Verification items for the finished model (mm, model axes). A direction names the side the tool comes from. Coordinates: 2 decimals unless noted, no trailing zeros. Loops run counter-clockwise (first coordinate to the right, second up) from the corner with the lowest first, then second, coordinate; pieces in that order, holes last. Notation, with made-up numbers: (31.5, 79.5) -> (83.5, 79.5) arc R17 cw to (83.5, 99.5) -> close; hole circle Ø4 at (-18, 59.25). An arc over 180 degrees is marked (long way). Write item = value, one per line.
```python
from build123d import *

# Parameters (mm, degrees)
BOSS_EXTRUDE1_DEPTH        = 10
CUT_EXTRUDE1_DEPTH         = 5
F_3_1_3_1_DIAMETER_HOLE2_D = 3.1
BOSS_EXTRUDE2_DEPTH        = 10
FILLET1_R                  = 3
FILLET2_R                  = 2
CUT_EXTRUDE6_DEPTH         = 2.5
SKETCH28_R                 = 3.5000000000000004
CUT_EXTRUDE7_DEPTH         = 2.5
SKETCH29_W                 = 2.5
SKETCH29_H                 = 3.5000000000000004
SKETCH30_R                 = 2.5000000000000004
CUT_EXTRUDE8_DEPTH         = 7.029807515


with BuildPart() as part:
    # Sketch1 → Boss-Extrude1 (new body)
    with BuildSketch(Plane(origin=(0, 0, 0), x_dir=(1, 0, 0), z_dir=(0, 1, 0))):
        with BuildLine():
            ThreePointArc((-207.41455152497886, 32.851237658448525), (-209.99999999999994, 2.572e-14), (-207.41455152497886, -32.85123765844857))
            Line((-207.41455152497886, -32.85123765844857), (-217.29143493093028, -34.41558230885091))
            ThreePointArc((-217.29143493093028, -34.41558230885091), (-220, 2.694e-14), (-217.29143493093028, 34.415582308850865))
            Line((-217.29143493093028, 34.415582308850865), (-207.41455152497886, 32.851237658448525))
        make_face()
        with BuildLine():
            ThreePointArc((-217.2914349309303, -34.415582308850915), (-219.99999999999997, -1.421e-14), (-217.2914349309303, 34.415582308850865))
            Line((-217.29143493093028, 34.41558230885082), (-219.26681161212053, 34.72845123893128))
            ThreePointArc((-219.26681161212053, 34.72845123893128), (-221.99999999999997, -2.665e-14), (-219.26681161212053, -34.72845123893134))
            Line((-219.26681161212053, -34.728451238931335), (-217.29143493093028, -34.41558230885088))
        make_face()
        with BuildLine():
            Line((-205.4391748437886, 32.538368728368056), (-207.41455152497886, 32.85123765844851))
            ThreePointArc((-207.41455152497886, 32.851237658448525), (-209.99999999999994, -2.132e-14), (-207.41455152497886, -32.85123765844859))
            Line((-207.41455152497886, -32.85123765844857), (-205.4391748437886, -32.53836872836811))
            ThreePointArc((-205.43917484378863, -32.53836872836813), (-207.99999999999997, -2.842e-14), (-205.43917484378863, 32.538368728368056))
        make_face()
    extrude(amount=BOSS_EXTRUDE1_DEPTH)

    # Sketch15 → Cut-Extrude1 (cut)
    with BuildSketch(Plane(origin=(0, 10, 0), x_dir=(1, 0, 0), z_dir=(0, 1, 0))):
        with BuildLine():
            Line((-219.7726097583591, 9.999999999999972), (-209.76176963403066, 9.999999999999972))
            ThreePointArc((-209.76176963403046, 9.999999999995824), (-208.90085088283388, 21.457737542154447), (-207.41455152497886, 32.851237658448504))
            Line((-207.41455152497886, 32.851237658448504), (-217.29143493093028, 34.41558230885091))
            ThreePointArc((-217.2914349309303, 34.41558230885091), (-218.8727368927212, 22.242415450882426), (-219.7726097583591, 10.000000000000421))
        make_face()
        with BuildLine():
            ThreePointArc((-207.4145515249789, -32.85123765844855), (-208.90085088283385, -21.457737542154504), (-209.76176963403046, -9.999999999995891))
            Line((-209.76176963403066, -10.000000000000028), (-219.77260975835907, -10.00000000000003))
            ThreePointArc((-219.7726097583591, -10.000000000000506), (-218.8727368927212, -22.242415450882447), (-217.2914349309303, -34.41558230885088))
            Line((-217.29143493093028, -34.41558230885086), (-207.41455152497886, -32.85123765844855))
        make_face()
    extrude(amount=-CUT_EXTRUDE1_DEPTH, mode=Mode.SUBTRACT)

    # Ø3.1 (3.1) Diameter Hole2 (through all)
    with Locations(Plane(origin=(0, 0, 0), x_dir=(-1, 0, 0), z_dir=(0, -1, 0))):
        with Locations((213.160645195, -28.063131327), (214.18186009, -18.738484691), (214.18186009, 18.738484691), (213.160645195, 28.063131327)):
            Hole(F_3_1_3_1_DIAMETER_HOLE2_D / 2)

    # Sketch19 → Boss-Extrude2 (add)
    with BuildSketch(Plane(origin=(0, 0, 0), x_dir=(1, 0, 0), z_dir=(0, 1, 0))):
        with BuildLine():
            Line((-205.06000872553298, -13.44034305679455), (-207.55465603362947, -13.603850879869908))
            ThreePointArc((-207.55465603362947, -13.603850879869908), (-207.99999999999994, 2.547e-14), (-207.55465603362947, 13.603850879869857))
            Line((-207.55465603362947, 13.603850879869857), (-205.06000872553298, 13.440343056794502))
            ThreePointArc((-205.06000872553298, 13.440343056794502), (-205.49999999999997, 2.517e-14), (-205.06000872553298, -13.44034305679455))
        make_face()
    extrude(amount=BOSS_EXTRUDE2_DEPTH)

    # Fillet1
    # the kernel refuses this fillet: 3 mm, written as the material it adds along each edge
    with BuildSketch(Plane(origin=(-207.5546560336295, 0, -13.60385087986986), x_dir=(0.07259195171826252, 0, -0.9973617240228008), z_dir=(0, 1, 0))) as fillet1_piece_1:
        with BuildLine():
            CenterArc((2.97605695844059, -2.9999221104362666), FILLET1_R, 89.58712595875737, 80.81905726138756)
            Line((0.01801487263020066, -2.4999350920302814), (-0.04114596908600657, -2.489935351662162))
            ThreePointArc((-0.04114596908600657, -2.489935351662162), (-0.05099100589383556, -1.2503999029582549), (-0.05999844220872477, -0.00043235694312724))
            Line((-0.05999844220872477, -0.00043235694312724), (-0.00043235694311419, 0.05999844220871681))
            ThreePointArc((-0.00043235694311419, 0.05999844220871681), (1.4988374027981592, 0.06540034308590705), (2.998107162539448, 0.05999844220873665))
            Line((2.998107162539448, 0.05999844220873665), (2.9976748055963345, 1e-17))
        make_face()
    extrude(amount=10)
    with BuildSketch(Plane(origin=(-207.5546560336295, 0, 13.60385087986991), x_dir=(0.07259195171826295, 0, 0.9973617240228008), z_dir=(0, 1, 0))) as fillet1_piece_2:
        with BuildLine():
            CenterArc((2.9760569584405734, 2.9999221104362666), FILLET1_R, 189.5938167798556, 80.819057261387)
            Line((0.01801487263018374, 2.4999350920302543), (-0.04114596908602352, 2.4899353516621354))
            ThreePointArc((-0.04114596908602352, 2.4899353516621354), (-0.05099100589383325, 1.2503999029582546), (-0.05999844220872477, 0.00043235694312726))
            Line((-0.05999844220872477, 0.00043235694312726), (-0.00043235694311422, -0.05999844220871681))
            ThreePointArc((-0.00043235694311422, -0.05999844220871681), (1.498837402798161, -0.06540034308590782), (2.9981071625394304, -0.05999844220873665))
            Line((2.9981071625394304, -0.05999844220873665), (2.9976748055963167, 0))
        make_face()
    extrude(amount=10)

    # Fillet2
    fillet2_edges = [part.edges().sort_by_distance(p)[0] for p in [
        (-219.26681161212053, 5, 34.72845123893134),
        (-219.26681161212053, 5, -34.728451238931285),
        (-205.43917484378863, 5, -32.538368728368056),
        (-205.43917484378863, 5, 32.53836872836813),
    ]]
    fillet(fillet2_edges, radius=FILLET2_R)

    # Sketch26 → Cut-Extrude6 (cut)
    with BuildSketch(Plane.XZ):
        with BuildLine():
            Line((-217.28245576049179, -34.41416014796698), (-207.40514475604385, -32.849747772616084))
            ThreePointArc((-207.40514475604385, -32.849747772616084), (-206.1055960612061, -32.057633278286005), (-205.73974688911358, -30.580329461983652))
            ThreePointArc((-205.73974688911358, -30.580329461983652), (-206.65676096006328, -23.600490450312087), (-207.33704896887454, -16.593616992039934))
            ThreePointArc((-207.33704896887454, -16.593616992039934), (-206.7787671555463, -14.597978692482226), (-205.06000872553278, -13.440343056794774))
            ThreePointArc((-205.06000872553278, -13.440343056794774), (-205.5, -6.609e-14), (-205.060008725533, 13.440343056794593))
            ThreePointArc((-205.060008725533, 13.440343056794593), (-206.77876715554575, 14.597978692481712), (-207.3370489688746, 16.593616992038744))
            ThreePointArc((-207.3370489688746, 16.593616992038744), (-206.6567609600633, 23.60049045031153), (-205.73974688911358, 30.580329461983624))
            ThreePointArc((-205.73974688911358, 30.580329461983624), (-206.10559606120609, 32.057633278286005), (-207.40514475604385, 32.84974777261609))
            Line((-207.40514475604385, 32.84974777261609), (-217.28245576049179, 34.41416014796698))
            ThreePointArc((-217.28245576049179, 34.41416014796698), (-218.7782378264501, 34.05145718237069), (-219.57346400594108, 32.7336814982928))
            ThreePointArc((-219.57346400594108, 32.7336814982928), (-221.99999999999994, 1.2577e-13), (-219.5734640059411, -32.733681498292746))
            ThreePointArc((-219.5734640059411, -32.733681498292746), (-218.7782378264501, -34.051457182370655), (-217.28245576049179, -34.41416014796698))
        make_face()
    extrude(amount=-CUT_EXTRUDE6_DEPTH, mode=Mode.SUBTRACT)

    # Sketch28 → Cut-Extrude7 (cut)
    with BuildSketch(Plane(origin=(-217.5, 0, 0), x_dir=(0, 0, -1), z_dir=(1, 0, 0))):
        with Locations((-2.082e-14, 10)):
            Circle(SKETCH28_R)
    extrude(amount=CUT_EXTRUDE7_DEPTH, mode=Mode.SUBTRACT)

    # Sketch29 → Cut-Revolve1 (revolve, cut)
    with BuildSketch(Plane(origin=(0, 10, 0), x_dir=(1, 0, 0), z_dir=(0, 1, 0))):
        with Locations((-206.72019248543083, -1.7500000000000002)):
            Rectangle(SKETCH29_W, SKETCH29_H)
    revolve(axis=Axis((-217.5, 10, 1.53e-15), (1, 0, -1.2e-16)), mode=Mode.SUBTRACT)

    # Sketch30 → Cut-Extrude8 (cut)
    with BuildSketch(Plane(origin=(-207.97019248543083, 0, 2.547e-14), x_dir=(-1.2e-16, 0, -1), z_dir=(1, 0, -1.2e-16))):
        with Locations((2.515e-14, 10)):
            Circle(SKETCH30_R)
    extrude(amount=-CUT_EXTRUDE8_DEPTH, mode=Mode.SUBTRACT)


solid = part.part
```
1) Tool access check on faces 5 (the face through (-217.5, 9, 0)), 6 (the face through (-207.97, 7, 0)), 7 (the face through (-212.75, 3.77, -18.14)), 8 (the face through (-212.367, 3.455, 33.636)), 9 (the face through (-206.646, 6.198, 23.698)). Record the directions out of +Z, -Z, +X, -X, +Y, -Y that give a thin tool (end or side, any length) a straight path to the whole face; none if there is none.
Ans:
face_5 = +Y
face_6 = +X, +Y
face_7 = +Y, -Y
face_8 = +Z, +X, +Y, -Y
face_9 = +X, +Y, -Y
2) Sectioned sample at A-A, the plane z = 0. Record the cut outline in (x, y).
Ans:
outline = (-222, 2.5) -> (-205.5, 2.5) -> (-205.5, 6.5) -> (-207.97, 6.5) -> (-207.97, 7.5) -> (-215, 7.5) -> (-215, 6.5) -> (-217.5, 6.5) -> (-217.5, 10) -> (-222, 10) -> close
3) Sectioned sample at B-B, the plane y = 3.75. Record the cut outline in (x, z), plus the area to 3 significant figures.
Ans:
outline = (-219.57, -32.73) arc R2 ccw to (-217.28, -34.41) -> (-207.41, -32.85) arc R2 ccw to (-205.74, -30.58) arc R208 cw to (-207.34, -16.59) arc R3 cw to (-205.06, -13.44) arc R205.5 cw to (-205.06, 13.44) arc R3 cw to (-207.34, 16.59) arc R208 cw to (-205.74, 30.58) arc R2 ccw to (-207.41, 32.85) -> (-217.28, 34.41) arc R2 ccw to (-219.57, 32.73) arc R222 ccw to start; hole circle Ø3.1 at (-214.18, -18.74); hole circle Ø3.1 at (-214.18, 18.74); hole circle Ø3.1 at (-213.16, -28.06); hole circle Ø3.1 at (-213.16, 28.06)
area = 983 mm2
4) Release check for a two-part mould opening along Z. For faces 1 (the face through (-218.855, 7.535, -22.413)), 2 (the face through (-213, 10, -3)), 3 (the face through (-218.76, 6.302, -34.064)), 4 (the face through (-211.4, 7.5, 0.1)) record: pulls with the +Z half, pulls with the -Z half, needs draft (parallel to the pull), parting line crosses it, or undercut.
Ans:
face_1 = undercut
face_2 = needs draft
face_3 = pulls with the -Z half
face_4 = undercut
5) Sectioned sample at C-C, the plane x = -216.5. Record the cut outline in (y, z).
Ans:
outline = (2.5, -34.29) -> (5, -34.29) -> (5, -10) -> (10, -10) -> (10, -3.5) arc R3.5 cw to (10, 3.5) -> (10, 10) -> (5, 10) -> (5, 34.29) -> (2.5, 34.29) -> close
6) Material ranges on line 1 (Z direction, x = -210, y = 9.75); line 2 (Z direction, x = -217, y = 6.25); line 3 (X direction, y = 9.25, z = -14.5), recorded low to high.
Ans:
line_1 = -10 to -2.49, 2.49 to 10
line_2 = -10 to 10
line_3 = -221.53 to -219.52, -209.5 to -206.7
7) Sectioned sample at D-D, the plane z = -23.5. Record the cut outline in (x, y).
Ans:
outline = (-220.75, 2.5) -> (-206.67, 2.5) -> (-206.67, 10) -> (-208.68, 10) -> (-208.68, 5) -> (-218.74, 5) -> (-218.74, 10) -> (-220.75, 10) -> close
8) Depth check by flat-ended pin: pin 1 Ø4 at (x, y) = (-216, 7.5) entering from -Z; pin 2 Ø2.5 at (x, z) = (-213.16, 28.06) entering from +Y; pin 3 Ø3 at (y, z) = (9, -1.5) entering from +X; pin 4 Ø5 at (x, z) = (-214.18, 18.74) entering from +Y. Enter the tip coordinate at first touch or a pass-through.
Ans:
pin_1 = -34.44
pin_2 = through
pin_3 = -207.97
pin_4 = 5
